Source: CAD feature listing. Evaluate the final solid. Frame: model axes, mm. Round coordinates to 2 decimals unless told otherwise and drop trailing zeros. Loops run counter-clockwise (first coordinate to the right, second up) from the corner with the lowest first, then second, coordinate; pieces in that order, holes last. Notation, with made-up numbers: M 37.25,33.5 L 56.25,33.5 A17 cw 56.25,65.5 Z; hole C -11.5,85.25 d5. An arc over 180 degrees is marked long. One line per item, written item: value.
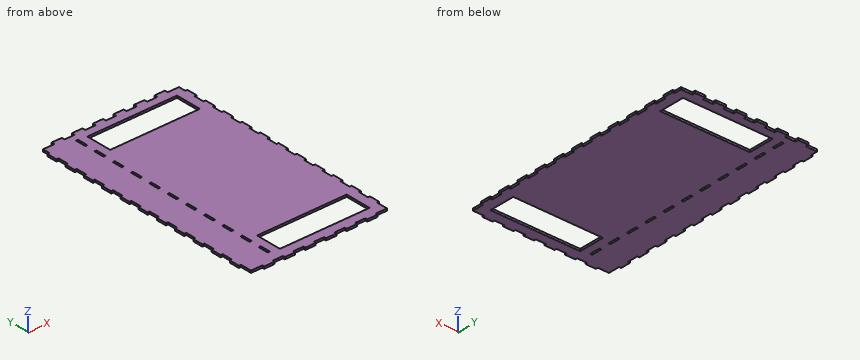
from build123d import *

# Parameters (mm, degrees)
SKETCH1_W           = 130
SKETCH1_H           = 227
SKETCH1_W_2         = 87
SKETCH1_H_2         = 25
BOSS_EXTRUDE1_DEPTH = 2
SKETCH2_W           = 10
SKETCH2_H           = 2
BOSS_EXTRUDE2_DEPTH = 3
LPATTERN1_COUNT     = 6
LPATTERN1_PITCH     = 20
SKETCH3_W           = 10
SKETCH3_H           = 2
BOSS_EXTRUDE3_DEPTH = 3
LPATTERN2_COUNT     = 6
LPATTERN2_PITCH     = 20
SKETCH4_W           = 2
SKETCH4_H           = 10
BOSS_EXTRUDE4_DEPTH = 3
LPATTERN3_COUNT     = 11
LPATTERN3_PITCH     = 20
SKETCH5_W           = 2
SKETCH5_H           = 10
BOSS_EXTRUDE5_DEPTH = 3
LPATTERN4_COUNT     = 11
LPATTERN4_PITCH     = 20
SKETCH6_W           = 3
SKETCH6_H           = 10
CUT_EXTRUDE1_DEPTH  = 3
LPATTERN5_COUNT     = 11
LPATTERN5_PITCH     = 20
ESQUISSE1_W         = 1
ESQUISSE1_H         = 210
ESQUISSE1_H_2       = 227
BOSS_EXTRU_1_DEPTH  = 2


with BuildPart() as part:
    # Sketch1 → Boss-Extrude1 (new body)
    with BuildSketch(Plane.XY):
        with Locations((65, 113.5)):
            Rectangle(SKETCH1_W, SKETCH1_H)
        with Locations((78.5, 20.5)):
            Rectangle(SKETCH1_W_2, SKETCH1_H_2, mode=Mode.SUBTRACT)
        with Locations((78.5, 206.5)):
            Rectangle(SKETCH1_W_2, SKETCH1_H_2, mode=Mode.SUBTRACT)
    extrude(amount=BOSS_EXTRUDE1_DEPTH)

    # Sketch2 → Boss-Extrude2 (add)
    with BuildSketch(Plane.XZ):
        with Locations((15, 1)):
            Rectangle(SKETCH2_W, SKETCH2_H)
    boss_extrude2 = extrude(amount=BOSS_EXTRUDE2_DEPTH)

    # LPattern1: Boss-Extrude2 ×6
    with Locations(*[(i * LPATTERN1_PITCH, 0, 0) for i in range(1, LPATTERN1_COUNT)]):
        add(boss_extrude2)

    # Sketch3 → Boss-Extrude3 (add)
    with BuildSketch(Plane(origin=(0, 227, 0), x_dir=(1, 0, 0), z_dir=(0, 1, 0))):
        with Locations((15, -1)):
            Rectangle(SKETCH3_W, SKETCH3_H)
    boss_extrude3 = extrude(amount=BOSS_EXTRUDE3_DEPTH)

    # LPattern2: Boss-Extrude3 ×6
    with Locations(*[(i * LPATTERN2_PITCH, 0, 0) for i in range(1, LPATTERN2_COUNT)]):
        add(boss_extrude3)

    # Sketch4 → Boss-Extrude4 (add)
    with BuildSketch(Plane(origin=(130, 0, 0), x_dir=(0, 0, -1), z_dir=(1, 0, 0))):
        with Locations((-1, 15)):
            Rectangle(SKETCH4_W, SKETCH4_H)
    boss_extrude4 = extrude(amount=BOSS_EXTRUDE4_DEPTH)

    # LPattern3: Boss-Extrude4 ×11
    with Locations(*[(0, i * LPATTERN3_PITCH, 0) for i in range(1, LPATTERN3_COUNT)]):
        add(boss_extrude4)

    # Sketch5 → Boss-Extrude5 (add)
    with BuildSketch(Plane.ZY):
        with Locations((1, 15)):
            Rectangle(SKETCH5_W, SKETCH5_H)
    boss_extrude5 = extrude(amount=BOSS_EXTRUDE5_DEPTH)

    # LPattern4: Boss-Extrude5 ×11
    with Locations(*[(0, i * LPATTERN4_PITCH, 0) for i in range(1, LPATTERN4_COUNT)]):
        add(boss_extrude5)

    # Sketch6 → Cut-Extrude1 (cut)
    with BuildSketch(Plane.XY.offset(2)):
        with Locations((26.5, 15)):
            Rectangle(SKETCH6_W, SKETCH6_H)
    cut_extrude1 = extrude(amount=-CUT_EXTRUDE1_DEPTH, mode=Mode.SUBTRACT)

    # LPattern5: Cut-Extrude1 ×11
    with Locations(*[(0, i * LPATTERN5_PITCH, 0) for i in range(1, LPATTERN5_COUNT)]):
        add(cut_extrude1, mode=Mode.SUBTRACT)

    # Esquisse1 → Boss.-Extru.1 (add)
    with BuildSketch(Plane.XY.offset(2)):
        Polygon((130, 0), (0, 0), (-1, 0), (-1, -1), (130, -1), align=None)
        with Locations((27.5, 115)):
            Rectangle(ESQUISSE1_W, ESQUISSE1_H)
        with Locations((-0.5, 113.5)):
            Rectangle(ESQUISSE1_W, ESQUISSE1_H_2)
        Polygon((130, 227), (130, 0), (130, -1), (131, -1), (131, 227), align=None)
    extrude(amount=-BOSS_EXTRU_1_DEPTH)


solid = part.part
1. Section query B-B (y = 26). Return the cut outline in (x, z).
Report:
outline: M -1,0 L 35,0 L 35,2 L -1,2 Z; M 122,0 L 131,0 L 131,2 L 122,2 Z
2. Ray query, line 1 (Y direction, x = 79.5, z = 0.9); line 2 (Y direction, x = 46, z = 1.05); line 3 (X direction, y = 214, z = 0.3). Return the intervals inside material, ascending. Write a range as [from, to].
Report:
line 1: y = [-3, 8], [33, 194], [219, 230]
line 2: y = [-1, 8], [33, 194], [219, 227]
line 3: x = [-3, 25], [27, 35], [122, 133]
3. Section query D-D (z = 1.5). Count the separate pieces of the cut face and the enclosed holes in it, and give its area (3 significant figures).
Report:
separate pieces: 1
enclosed holes: 13
area: 26,300 mm2
4. Section query C-C (x = 103.5). Return the cut outline in (y, z), and give its area (3 significant figures).
Report:
outline: M -1,0 L 8,0 L 8,2 L -1,2 Z; M 33,0 L 194,0 L 194,2 L 33,2 Z; M 219,0 L 227,0 L 227,2 L 219,2 Z
area: 356 mm2
5. Pin query (flat end, axial travel): pin 1 (1 mm diameter, centred on x = 82, y = 99, fed in from -Z); pin 2 (0.6 mm diameter, centred on x = 25.5, z = 1, fed in from +Y); pin 3 (1 mm diameter, centred on x = 132, z = 0.5, fed in from +Y); pin 4 (0.6 mm diameter, centred on x = 7, z = 1, fed in from -Y). Return the tip coordinate at first contact, or that it passes through.
Report:
pin 1: stops at z = 0
pin 2: stops at y = 227
pin 3: stops at y = 220
pin 4: stops at y = -1
6. Section query A-A (x = 77). Return the cut outline in (y, z).
Report:
outline: M -3,0 L 8,0 L 8,2 L -3,2 Z; M 33,0 L 194,0 L 194,2 L 33,2 Z; M 219,0 L 230,0 L 230,2 L 219,2 Z
